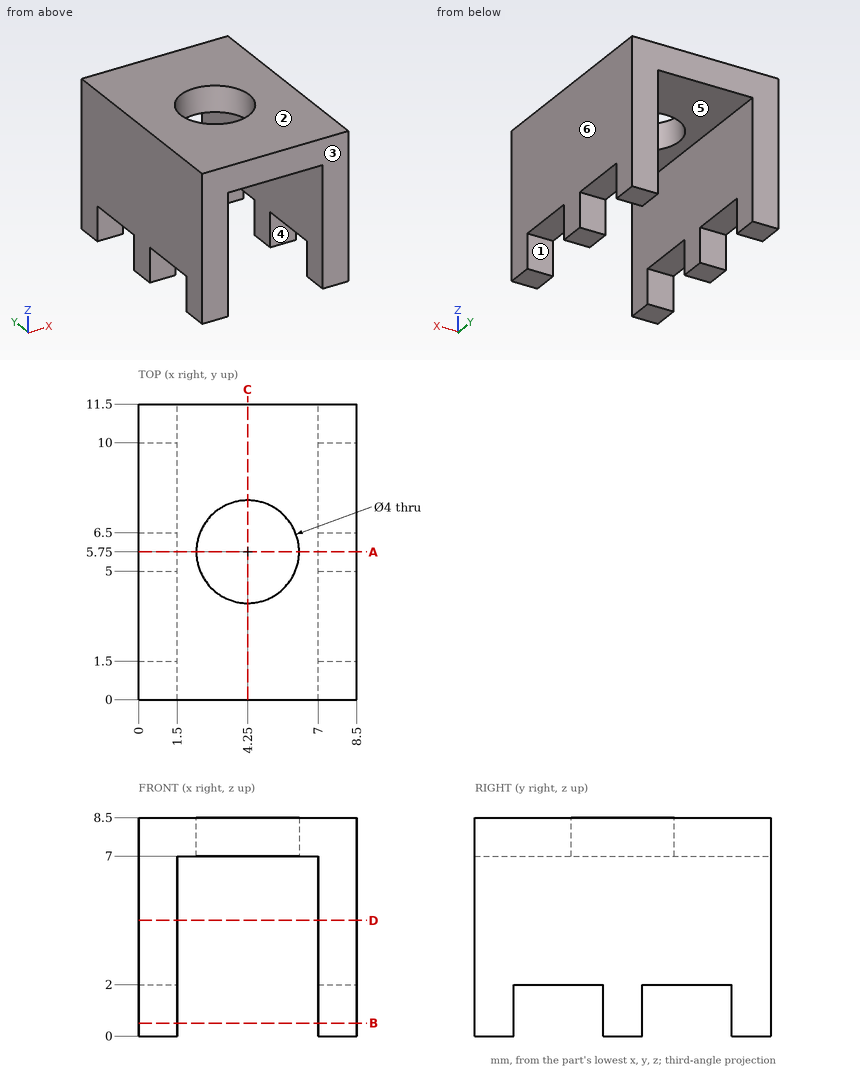
Study the drawing (mm; zero at the part's minimum x, y, z) and answer. A direction names the side the tool comes from. Give positions to 0.01 mm unless a question says otherwise; leave off trailing zeros. Order: outer loops, then holes, each group sorted by start corner. A loop starts at its lowest first (then second) coordinate and runs counter-clockwise, first axis right, second up. Notation, with made-up numbers: M 69.25,31.25 L 107.25,31.25 A21 cw 107.25,68.25 Z; hole C -10,16 d7. An arc over 180 degrees is marked long. Put each result on its own line as item: value. Start each with the question number.
Item 1: The part is cut by section C-C, the plane x = 4.25. Determine the outline of the cut face in (y, z), and give its area (4 significant figures).
Item 2: The part is cut by section A-A, the plane y = 5.75. Determine the outline of the cut face in (x, z).
Item 3: Find the intervals of material crossed by line 1 along Y through (x, z) = (4.25, 7.45); line 2 along X through (y, z) = (6, 1.75); line 3 along Z through (x, y) = (2.25, 4.5), in increasing order.
Item 4: For a pull along Y with two mould halves and no side action, classify the marked faces 1, 2 and 3 as +Y half, -Y half, draft (parallel to the pull), parting line (faces both ways), or undercut.
Item 5: The part is cut by section B-B, the plane z = 0.5. Determine the outline of the cut face in (x, y), and give its area (3 significant figures).
Item 6: A flat-ended cylindrical pin translates along its axis: P1, Ø1.6, axis at x = 0.5, y = 8, coming from the -Z side. Find the tip coordinate at first contact, or state that the pin passes through.
Item 7: Which of the six approach directions +Z, -Z, +X, -X, +Y, -Y give full straight-line access (tool end or side, diameter ignored) to the marked faces 4, 5 and 6?
Item 8: The part is cut by section D-D, the plane z = 4.5. Determine the outline of the cut face in (x, y).
Answer key:
1. outline: M 0,7 L 3.75,7 L 3.75,8.5 L 0,8.5 Z; M 7.75,7 L 11.5,7 L 11.5,8.5 L 7.75,8.5 Z
1. area: 11.25 mm²
2. outline: M 0,0 L 1.5,0 L 1.5,7 L 2.25,7 L 2.25,8.5 L 0,8.5 Z; M 6.25,7 L 7,7 L 7,0 L 8.5,0 L 8.5,8.5 L 6.25,8.5 Z
3. line 1: y = 0 to 3.75, 7.75 to 11.5
3. line 2: x = 0 to 1.5, 7 to 8.5
3. line 3: z = 7 to 8.5
4. face 1: undercut
4. face 2: draft
4. face 3: -Y half
5. outline: M 0,0 L 1.5,0 L 1.5,1.5 L 0,1.5 Z; M 0,5 L 1.5,5 L 1.5,6.5 L 0,6.5 Z; M 0,10 L 1.5,10 L 1.5,11.5 L 0,11.5 Z; M 7,0 L 8.5,0 L 8.5,1.5 L 7,1.5 Z; M 7,5 L 8.5,5 L 8.5,6.5 L 7,6.5 Z; M 7,10 L 8.5,10 L 8.5,11.5 L 7,11.5 Z
5. area: 13.5 mm²
6. P1: stops at z = 2
7. face 4: -Z, +X, -X
7. face 5: -Z, +Y, -Y
7. face 6: +Z, -Z, +X, +Y, -Y
8. outline: M 0,0 L 1.5,0 L 1.5,11.5 L 0,11.5 Z; M 7,0 L 8.5,0 L 8.5,11.5 L 7,11.5 Z
